Can you work these out from the model? Positions are in its coordinate system, mm. Face numbers are marked on the shaded views. Coordinates: 2 decimals unless noted, no trailing zeros. Order: outer loops, then holes, each group sorted by start corner. A loop starts at its lowest first (then second) coordinate and runs counter-clockwise, first axis right, second up. Notation, with made-up numbers: (38, 49.25) -> (96, 49.25) arc R16 ccw to (96, 58.25) -> close; hole circle Ø11 at (34, -21.75). An arc over 180 degrees is marked (long way). Use a Markdown table: item, result. Add a question column.
1. Suppose I cut it at A-A, the plane x = 0. List the corners of the cut face in (y, z) for me.
2. For pin 1 Ø1 at (x, z) = (-11.5, 3) entering from +Y; pin 2 Ø10 at (y, z) = (-9.5, 1) entering from -X; pin 3 Ø6 at (y, z) = (-8, 5.5) entering from -X; pin 4 Ø8 at (x, z) = (0, 0) entering from -Y, each with a flat end and sliding along its axis, tell me the tip position at first contact or that it passes through.
3. Suppose I cut it at D-D, the plane z = 2.5. List the corners of the cut face in (x, y) for me, then the cut area to 3 significant figures.
4. We'd pull the mould along X, two halves only. Please class the marked faces 1, 2 and 3: pulls with the +X half, pulls with the -X half, needs draft (parallel to the pull), parting line crosses it, or undercut.
5. Suppose I cut it at B-B, the plane y = 0. List the corners of the cut face in (x, z) for me, then the cut area to 3 significant figures.
6. If I drill on line 1 along X through (y, z) = (0.5, 3.25); line 2 along Z through (x, y) = (0, -18.5); line 3 along X through (y, z) = (6.5, -6.5), over which ranges is the centre line in solid material (lowest first)? Write a range as from..to.
7. Suppose I cut it at C-C, the plane z = -5.25. List the corners of the cut face in (x, y) for me, then the cut area to 3 significant figures.
Autodesk Fusion 360 part; units mm, degrees
sketch "Sketch1" plane through (0, 0, 0) normal (0, 0, 1) x (1, 0, 0)
  circle A0 centre (0, 0) radius 11
  circle A1 centre (0, 0) radius 21
  dimension "d1" = 22
  dimension "d2" = 42
extrude "Extrude1" add sketch "Sketch1" along normal mid plane 18
chamfer "Chamfer1" distance 2 angle 45 2 edges at (-19.5789, -7.5939, 9) (-19.5789, 7.5939, -9)
sketch "Sketch2" plane through (0, 0, 0) normal (0, 1, 0) x (1, 0, 0)
  circle A0 centre (0, 0) radius 3
  dimension "d6" = 6
extrude "Extrude2" cut sketch "Sketch2" against normal blind 32
thread "Thread1" thread offset 0 thread length 10
thread "Thread2" thread offset 0 thread length 10
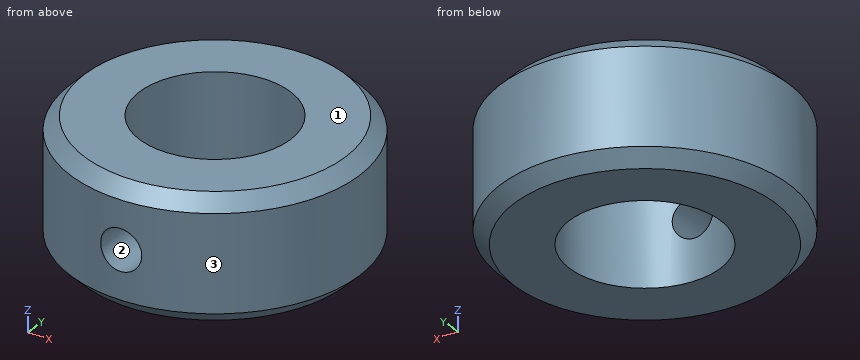
Worked out:
| question | item | result |
|---|---|---|
| 1 | outline | (-21, -7) -> (-19, -9) -> (-11, -9) -> (-11, -3) -> (-21, -3) -> close; (-21, 3) -> (-11, 3) -> (-11, 9) -> (-19, 9) -> (-21, 7) -> close; (11, -9) -> (19, -9) -> (21, -7) -> (21, 7) -> (19, 9) -> (11, 9) -> close |
| 2 | pin 1 | stops at y = 17.89 |
| 2 | pin 2 | stops at x = -20.51 |
| 2 | pin 3 | stops at x = -20.4 |
| 2 | pin 4 | stops at y = -21 |
| 3 | outline | (-1.66, -20.93) -> (-1.66, -10.87) arc R11 cw (long way) to (1.66, -10.87) -> (1.66, -20.93) arc R21 ccw (long way) to start |
| 3 | area | 972 mm² |
| 4 | face 1 | needs draft |
| 4 | face 2 | undercut |
| 4 | face 3 | parting line crosses it |
| 5 | outline | (-21, -7) -> (-19, -9) -> (-11, -9) -> (-11, 9) -> (-19, 9) -> (-21, 7) -> close; (11, -9) -> (19, -9) -> (21, -7) -> (21, 7) -> (19, 9) -> (11, 9) -> close |
| 5 | area | 352 mm² |
| 6 | line 1 | x = -20.99..-10.99, 10.99..20.99 |
| 6 | line 2 | z = -9..-3, 3..9 |
| 6 | line 3 | x = -19.97..-8.87, 8.87..19.97 |
| 7 | outline | circle Ø42 at (0, 0); hole circle Ø22 at (0, 0) |
| 7 | area | 1,010 mm² |
